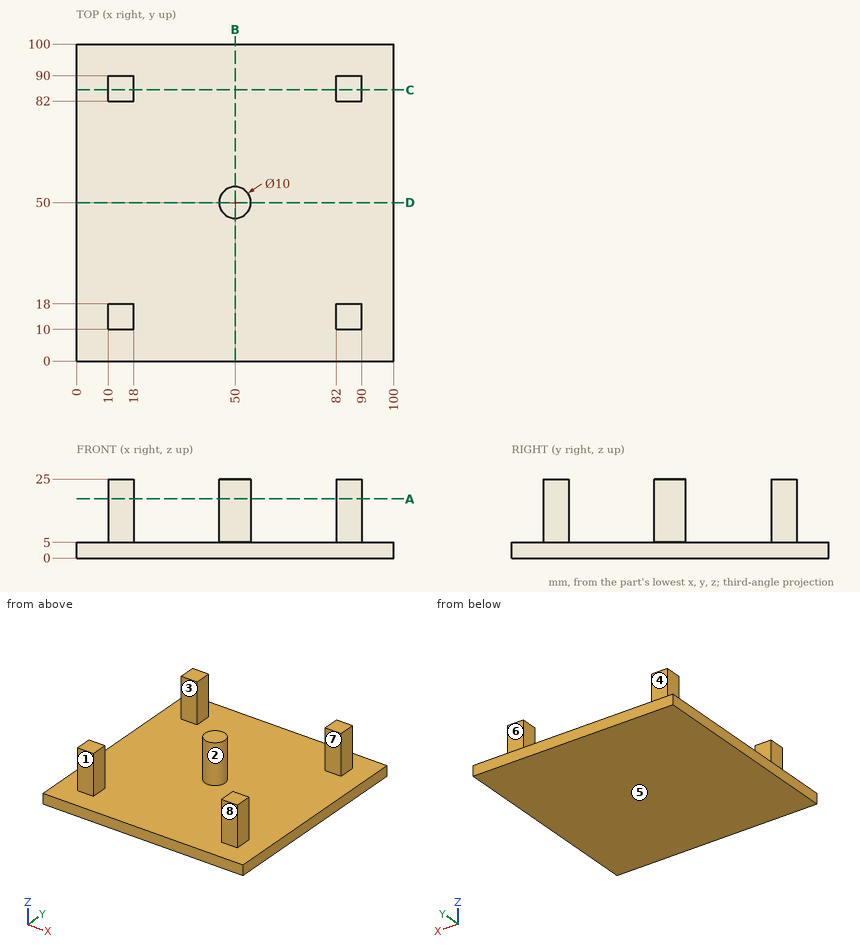
Part print with two shaded views. Sizes in mm from the minimum x, y, z corner. A direction names the side the tool comes from. Give positions to 0.01 mm unless a question says otherwise; leave off trailing zeros. Order: outer loops, then holes, each group sorted by start corner. A loop starts at its lowest first (then second) coordinate and runs counter-clockwise, first axis right, second up. Notation, with made-up numbers: M -31,-7 L 0,-7 A19 ccw 0,12 Z; hole C -4,-10 d5. An arc over 180 degrees is marked long. Use one line per item in the form item = value.
1) Saw through at C-C (y = 85.5). Give the cut face in (x, z), plus the area to 3 significant figures.
Calculated:
outline = M 0,0 L 100,0 L 100,5 L 90,5 L 90,25 L 82,25 L 82,5 L 18,5 L 18,25 L 10,25 L 10,5 L 0,5 Z
area = 820 mm2
2) Drop flat-ended pins along their axis: pin 1 (6.5 mm diameter, centred on x = 14, z = 17, fed in from -Y); pin 2 (10 mm diameter, centred on x = 84, y = 78, fed in from -Z); pin 3 (6.5 mm diameter, centred on y = 12.5, z = 15, fed in from -X); pin 4 (8 mm diameter, centred on x = 80.5, z = 9.5, fed in from +Y). Give the stop position or say it passes through.
Calculated:
pin_1 = 10
pin_2 = 0
pin_3 = 10
pin_4 = 90
3) Tool access for the marked faces 5, 6, 7 and 8: list every direction of +Z, -Z, +X, -X, +Y, -Y with a clear straight run to the whole face (end or side of a thin tool).
Calculated:
face_5 = -Z, +X, -X, +Y, -Y
face_6 = +Z, +X, -X, +Y
face_7 = +Z, +X, -X
face_8 = +Z, +X, -X, -Y
4) Probe probe 1 along Z at (x, y) = (76, 41); probe 2 along Y at (x, z) = (16.5, 8.25). List the from-to ranges inside material, lowest first.
Calculated:
probe_1 = 0 to 5
probe_2 = 10 to 18, 82 to 90
5) Two-plate mould, pull along Y, no slides. Class the marked faces 1, 2, 3 and 4: released by +Y, released by -Y, zero draft, split by the parting line, or undercut.
Calculated:
face_1 = released by -Y
face_2 = split by the parting line
face_3 = undercut
face_4 = released by +Y
6) Saw through at A-A (z = 18.75). Give the cut face in (x, y).
Calculated:
outline = M 10,10 L 18,10 L 18,18 L 10,18 Z; M 10,82 L 18,82 L 18,90 L 10,90 Z; C 50,50 d10; M 82,10 L 90,10 L 90,18 L 82,18 Z; M 82,82 L 90,82 L 90,90 L 82,90 Z
7) Saw through at B-B (x = 50). Give the cut face in (y, z), plus the area to 3 significant figures.
Calculated:
outline = M 0,0 L 100,0 L 100,5 L 55,5 L 55,25 L 45,25 L 45,5 L 0,5 Z
area = 700 mm2
